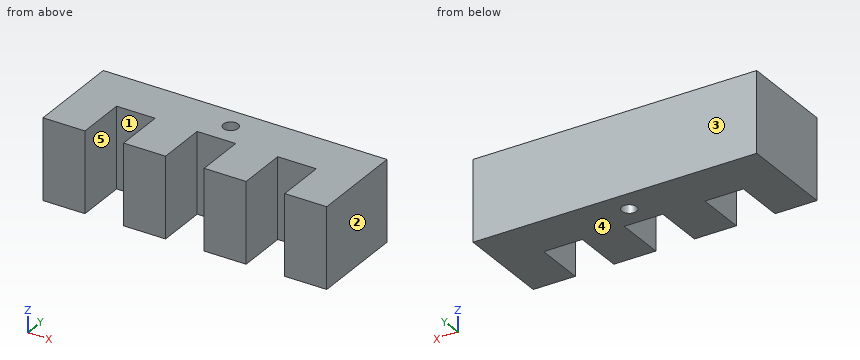
from build123d import *

# Parameters (mm, degrees)
F0_R     = 1.651
F1_DEPTH = 18.034


with BuildPart() as f1:
    # F0 (on Top) → F1 (new body)
    with BuildSketch(Plane.XY):
        Polygon((-54.102, 10.16), (-54.102, 0), (-54.102, -11.176), (-44.704, -11.176), (-44.704, 0), (-36.068, 0), (-36.068, -11.176), (-26.67, -11.176), (-26.67, 0), (-18.034, 0), (-18.034, -11.176), (-8.636, -11.176), (-8.636, 0), (0, 0), (0, -11.176), (9.398, -11.176), (9.398, 10.16), align=None)
        with Locations((-22.352, 5.08)):
            Circle(F0_R, mode=Mode.SUBTRACT)
    extrude(amount=F1_DEPTH)


solid = f1.part
Verification items for the finished model (mm, model axes). Face numbers are marked on the shaded views. A direction names the side the tool comes from. Give positions to 0.01 mm unless a question says otherwise; leave off trailing zeros. Order: outer loops, then holes, each group sorted by start corner. A loop starts at its lowest first (then second) coordinate and runs counter-clockwise, first axis right, second up. Notation, with made-up numbers: M -29,60.5 L 4,60.5 A22 cw 4,99.5 Z; hole C 80.5,-2 d1. An arc over 180 degrees is marked long. Answer as a JSON object with one key per item and string values. Group by question number.
1) Cross-section at D-D (y = -3). Enter the section's corners in (x, z).
2) Cross-section at C-C (z = 13.25). Enter the section's corners in (x, y).
3) Depth check by flat-ended pin: pin 1 Ø9.5 at (x, z) = (-42, 12.5) entering from -Y; pin 2 Ø2.5 at (x, z) = (-23.5, 11.5) entering from -Y. Enter the tip coordinate at first touch or a pass-through.
4) Access from +Z, -Z, +X, -X, +Y, -Y to the whole of each face (thin tool, end or side, straight path). Record for the marked faces 4 and 5.
5) Mould release check, pull along X, two halves, no side actions. Record for the marked faces 1, 2 and 3: released by +X, released by -X, zero draft, split by the parting line, or undercut.
6) Cross-section at A-A (y = 5.08). Enter the section's corners in (x, z), then the cut area to 3 significant figures.
7) Cross-section at B-B (x = -23). Enter the section's corners in (y, z).
8) Scan lines: line 1 along X through (y, z) = (-8.75, 9.25); line 2 along X through (y, z) = (5, 9.25); line 3 along Y through (x, z) = (-5, 12.5). Record each from-to range of solid material in increasing order. Write a range as [from, to].
Result sheet:
{
 "1": {"outline": "M -54.1,0 L -44.7,0 L -44.7,18.03 L -54.1,18.03 Z; M -36.07,0 L -26.67,0 L -26.67,18.03 L -36.07,18.03 Z; M -18.03,0 L -8.64,0 L -8.64,18.03 L -18.03,18.03 Z; M 0,0 L 9.4,0 L 9.4,18.03 L 0,18.03 Z"},
 "2": {"outline": "M -54.1,-11.18 L -44.7,-11.18 L -44.7,0 L -36.07,0 L -36.07,-11.18 L -26.67,-11.18 L -26.67,0 L -18.03,0 L -18.03,-11.18 L -8.64,-11.18 L -8.64,0 L 0,0 L 0,-11.18 L 9.4,-11.18 L 9.4,10.16 L -54.1,10.16 Z; hole C -22.35,5.08 d3.3"},
 "3": {"pin 1": "stops at y = -11.18", "pin 2": "stops at y = 0"},
 "4": {"face 4": "-Z, +X, -X, +Y, -Y", "face 5": "+Z, -Z, -Y"},
 "5": {"face 1": "undercut", "face 2": "released by +X", "face 3": "zero draft"},
 "6": {"outline": "M -54.1,0 L -24,0 L -24,18.03 L -54.1,18.03 Z; M -20.7,0 L 9.4,0 L 9.4,18.03 L -20.7,18.03 Z", "area": "1,090 mm2"},
 "7": {"outline": "M 0,0 L 3.56,0 L 3.56,18.03 L 0,18.03 Z; M 6.6,0 L 10.16,0 L 10.16,18.03 L 6.6,18.03 Z"},
 "8": {"line 1": "x = [-54.1, -44.7], [-36.07, -26.67], [-18.03, -8.64], [0, 9.4]", "line 2": "x = [-54.1, -24], [-20.7, 9.4]", "line 3": "y = [0, 10.16]"}
}
